Can you work these out from the drawing? Everything is in mm from the part's minimum corner. A direction names the side the tool comes from. Round coordinates to 2 decimals unless told otherwise and drop trailing zeros. Write each loop counter-clockwise with the first axis right and the second up, starting at its lowest first coordinate (ties: lowest second). Pieces come first, ordered by that corner, then holes. Notation, with made-up numbers: (58, 81) -> (109, 81) arc R22 cw to (109, 93) -> close; hole circle Ø1 at (-11.5, 64). An arc over 180 degrees is marked (long way). One line per question, with ' | ' between items. Start each with the question number.
1. Imagine slicing it at A-A, the plane y = 41. List the corners of the cut face in (x, z) for me.
2. For the marked faces 1 and 2, which set-ups out of +Z, -Z, +X, -X, +Y, -Y let a thin tool reach every point of the face, with its end or its side?
3. For pin 1 Ø11 at (y, z) = (21, 16) entering from -X; pin 2 Ø8 at (x, z) = (25, 13) entering from -Y; pin 3 Ø1 at (x, y) = (26, 15) entering from +Z; pin 4 Ø8 at (x, y) = (42.5, 44) entering from -Z, each with a flat end and sliding along its axis, tell me the tip position at first contact or that it passes through.
4. If I drill on line 1 along Z through (x, y) = (43.5, 43); line 2 along Y through (x, z) = (22, 3.5); line 3 along X through (y, z) = (45.5, 16), over which ranges is the centre line in solid material (lowest first)? Write a range as [from, to].
5. Imagine slicing it at B-B, the plane y = 47. List the corners of the cut face in (x, z) for me, and give its area (3 significant figures).
6. Imagine slicing it at D-D, the plane z = 20.75. List the corners of the cut face in (x, y) for me.
7. Thinking about a two-plate mould opening in Z: for the marked faces 3, 4 and 5, which applies, released by +Z, released by -Z, zero draft, split by the parting line, or undercut?
8. Imagine slicing it at C-C, the plane x = 43. List the corners of the cut face in (y, z) for me, and give its area (3 significant figures).
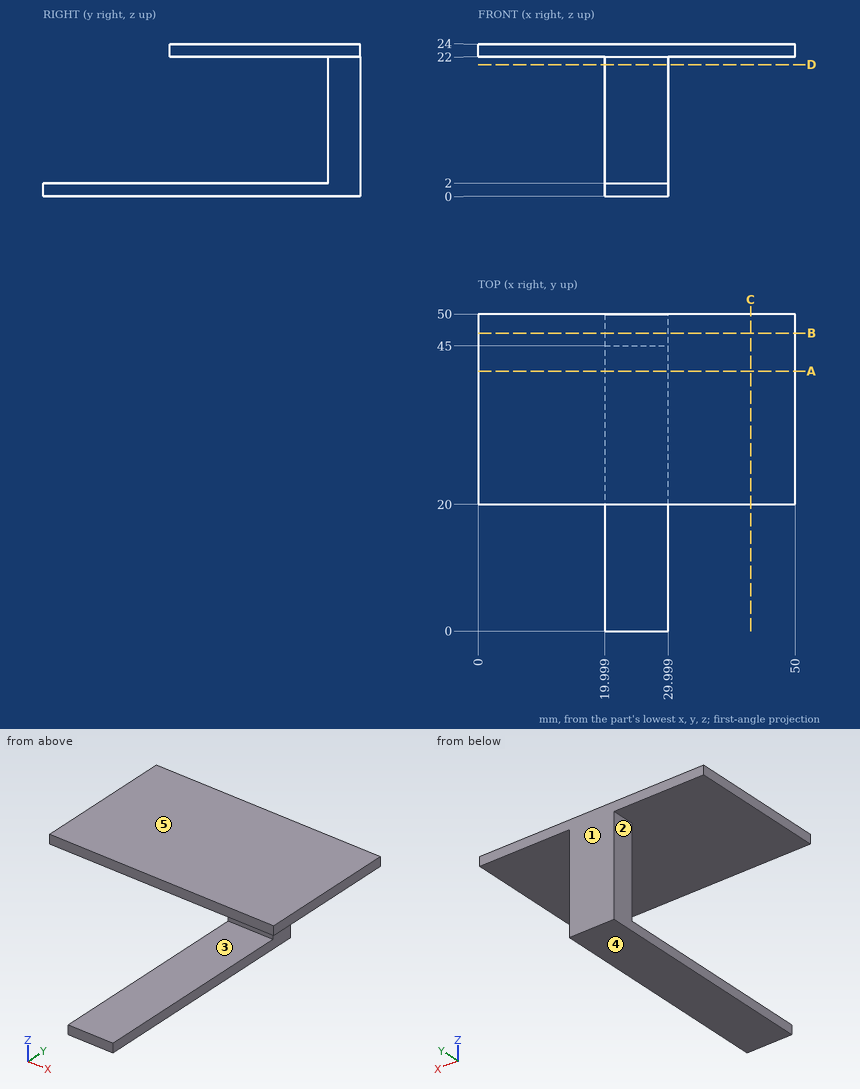
Geometry results:
1) outline: (0, 22) -> (50, 22) -> (50, 24) -> (0, 24) -> close; (20, 0) -> (30, 0) -> (30, 2) -> (20, 2) -> close
2) face 1: +Z, -Z, +X, -X, +Y | face 2: -Z, -X, +Y, -Y
3) pin 1: passes through | pin 2: stops at y = 45 | pin 3: stops at z = 2 | pin 4: stops at z = 22
4) line 1: z = [22, 24] | line 2: y = [45, 50] | line 3: x = [20, 30]
5) outline: (0, 22) -> (20, 22) -> (20, 0) -> (30, 0) -> (30, 22) -> (50, 22) -> (50, 24) -> (0, 24) -> close | area: 320 mm2
6) outline: (20, 45) -> (30, 45) -> (30, 50) -> (20, 50) -> close
7) face 3: undercut | face 4: released by -Z | face 5: released by +Z
8) outline: (20, 22) -> (50, 22) -> (50, 24) -> (20, 24) -> close | area: 60.0 mm2
